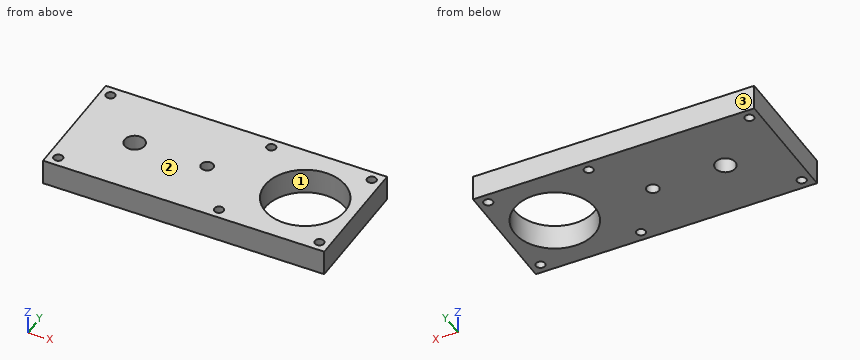
```python
from build123d import *

# Parameters (mm, degrees)
SKETCH1_W             = 70
SKETCH1_H             = 30
BOSS_EXTRUDE1_DEPTH   = 6.35
F_2_CLEARANCE_HOLE1_D = 2.2606
SKETCH4_R             = 10
SKETCH4_R_2           = 2.4892
SKETCH4_R_3           = 1.525
CUT_EXTRUDE1_DEPTH    = 77.422002722


with BuildPart() as part:
    # Sketch1 → Boss-Extrude1 (new body)
    with BuildSketch(Plane.XY):
        with Locations((35, 15)):
            Rectangle(SKETCH1_W, SKETCH1_H)
    extrude(amount=BOSS_EXTRUDE1_DEPTH)

    # #2 Clearance Hole1 (through all)
    with Locations(Plane.XY.offset(6.35)):
        with Locations((2.5, 27.5), (42.5, 27.5), (67.5, 27.5), (67.5, 2.5), (42.5, 2.5), (2.5, 2.5)):
            Hole(F_2_CLEARANCE_HOLE1_D / 2)

    # Sketch4 → Cut-Extrude1 (cut, through all)
    with BuildSketch(Plane.XY.offset(6.35)):
        with Locations((57.45, 15)):
            Circle(SKETCH4_R)
        with Locations((15, 15)):
            Circle(SKETCH4_R_2)
        with Locations((33.05, 15)):
            Circle(SKETCH4_R_3)
    extrude(amount=-CUT_EXTRUDE1_DEPTH, mode=Mode.SUBTRACT)


solid = part.part
```
Design review of the part built by this model. Coordinates are the model's own, in mm. Face numbers are marked on the shaded views. Coordinates: 2 decimals unless noted, no trailing zeros. Order: outer loops, then holes, each group sorted by start corner. A loop starts at its lowest first (then second) coordinate and runs counter-clockwise, first axis right, second up. Notation, with made-up numbers: (4.25, -16) -> (8.25, -16) arc R16 cw to (8.25, 4) -> close; hole circle Ø1 at (73.5, 42.5). An arc over 180 degrees is marked (long way). One line per item, written item: value. Start each with the question number.
Q1. For probe 1 along Y at (x, z) = (42.5, 2.75); probe 2 along Y at (x, z) = (15, 3.25); probe 3 along X at (y, z) = (1.5, 5.5), list the stretches that pass through material, from the lowest coordinate up.
Q2. Take a section at A-A, the plane y = 9. State the section outline as (x, z) points.
Q3. Take a section at D-D, the plane x = 42.5. State the section outline as (y, z) points, then the cut area to 3 significant figures.
Q4. Mouldability with a two-part tool opening along Y and no side actions: class the marked faces 1, 2 and 3 as pulls with the +Y half, pulls with the -Y half, needs draft (parallel to the pull), parting line crosses it, or undercut.
Q5. Take a section at C-C, the plane z = 2.25. Give the number of separate pieces and of enclosed holes in the cut face, then the cut area to 3 significant figures.
Q6. Take a section at B-B, the plane x = 33.05. State the section outline as (y, z) points (3 decimals), then the cut area to 3 significant figures.
Values follow:
1. probe 1: y = 0 to 1.37, 3.63 to 26.37, 28.63 to 30
1. probe 2: y = 0 to 12.51, 17.49 to 30
1. probe 3: x = 0 to 1.97, 3.03 to 41.97, 43.03 to 66.97, 68.03 to 70
2. outline: (0, 0) -> (49.45, 0) -> (49.45, 6.35) -> (0, 6.35) -> close; (65.45, 0) -> (70, 0) -> (70, 6.35) -> (65.45, 6.35) -> close
3. outline: (0, 0) -> (1.37, 0) -> (1.37, 6.35) -> (0, 6.35) -> close; (3.63, 0) -> (26.37, 0) -> (26.37, 6.35) -> (3.63, 6.35) -> close; (28.63, 0) -> (30, 0) -> (30, 6.35) -> (28.63, 6.35) -> close
3. area: 162 mm2
4. face 1: undercut
4. face 2: needs draft
4. face 3: pulls with the +Y half
5. separate pieces: 1
5. enclosed holes: 9
5. area: 1,730 mm2
6. outline: (0, 0) -> (13.475, 0) -> (13.475, 6.35) -> (0, 6.35) -> close; (16.525, 0) -> (30, 0) -> (30, 6.35) -> (16.525, 6.35) -> close
6. area: 171 mm2
